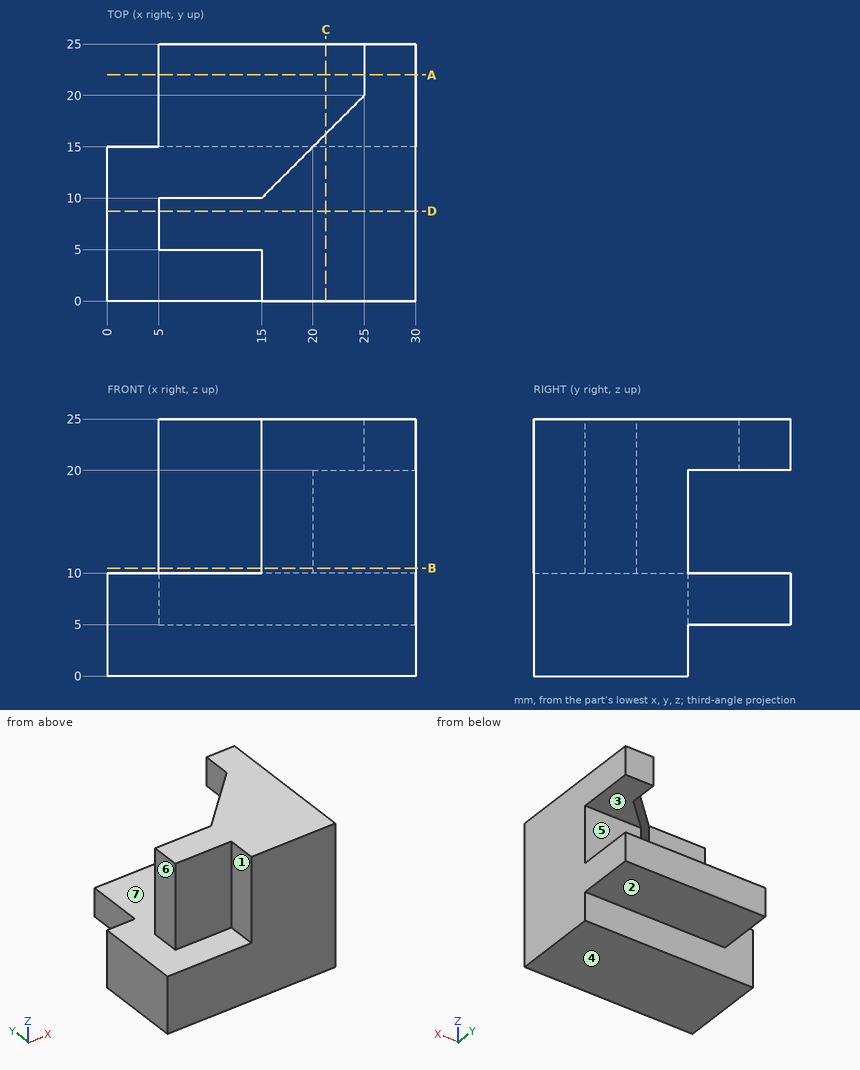
Could you check a few things on this drawing? It's one solid part, dimensions in mm from its lowest x, y, z. A direction names the side the tool comes from. Coordinates: 2 decimals unless noted, no trailing zeros. Write each loop counter-clockwise with the first axis right and the second up, starting at its lowest first coordinate (ties: lowest second). Pieces come first, ordered by that corner, then holes. Notation, with made-up numbers: (55, 50) - (85, 50) arc R17 ccw to (85, 67) - close; hole circle Ø1 at (49.25, 14). An arc over 180 degrees is marked (long way). Return JSON: item names as keys, results as strings. Group by question number.
Item 1: I'm going to push flat-ended pins straight in: pin 1 Ø8 at (x, z) = (9, 19) entering from +Y; pin 2 Ø4 at (x, z) = (4.5, 13) entering from -Y; pin 3 Ø5 at (x, z) = (23.5, 14) entering from +Y. Where does each tip first touch, or does it pass through?
Item 2: If we section it at B-B (z = 10.5): Write out the boundary of the cut face in (x, y), then the cut area to 4 significant figures.
Item 3: If we section it at A-A (y = 22): Write out the boundary of the cut face in (x, z).
Item 4: Please list where these lines run through material, in increasing order: probe 1 along Y at (x, z) = (6.25, 13); probe 2 along X at (y, z) = (6.75, 12.75); probe 3 along Z at (x, y) = (11.5, 14).
Item 5: Which directions (+Z, -Z, +X, -X, +Y, -Y) give clear straight access to the entire face, cutting with the end or side of a thin tool? Please do the marked faces 1, 2 and 3.
Item 6: We'd pull the mould along Z, two halves only. Please class the marked faces 4, 5, 6 and 7: pulls with the +Z half, pulls with the -Z half, needs draft (parallel to the pull), parting line crosses it, or undercut.
Item 7: If we section it at D-D (y = 8.75): Write out the boundary of the cut face in (x, z), then the cut area to 3 significant figures.
Item 8: If we section it at C-C (x = 21.25): Write out the boundary of the cut face in (y, z), then the cut area to 3 significant figures.
Return value:
{
 "1": {"pin 1": "stops at y = 10", "pin 2": "stops at y = 5", "pin 3": "stops at y = 15"},
 "2": {"outline": "(5, 5) - (15, 5) - (15, 0) - (30, 0) - (30, 15) - (20, 15) - (15, 10) - (5, 10) - close", "area": "262.5 mm^2"},
 "3": {"outline": "(5, 5) - (30, 5) - (30, 10) - (5, 10) - close; (25, 20) - (30, 20) - (30, 25) - (25, 25) - close"},
 "4": {"probe 1": "y = 5 to 10", "probe 2": "x = 5 to 30", "probe 3": "z = 0 to 10"},
 "5": {"face 1": "+Z, -X, -Y", "face 2": "-Z, +X, -X, +Y", "face 3": "+X, -X, +Y"},
 "6": {"face 4": "pulls with the -Z half", "face 5": "undercut", "face 6": "needs draft", "face 7": "undercut"},
 "7": {"outline": "(0, 0) - (30, 0) - (30, 25) - (5, 25) - (5, 10) - (0, 10) - close", "area": "675 mm^2"},
 "8": {"outline": "(0, 0) - (15, 0) - (15, 5) - (25, 5) - (25, 10) - (15, 10) - (15, 20) - (16.25, 20) - (16.25, 25) - (0, 25) - close", "area": "431 mm^2"}
}
